Build history of the part. All positions in model axes, mm. Face numbers are marked on the shaded views. A direction names the side the tool comes from. Coordinates: 2 decimals unless noted, no trailing zeros. Order: outer loops, then holes, each group sorted by start corner. A loop starts at its lowest first (then second) coordinate and runs counter-clockwise, first axis right, second up. Notation, with made-up numbers: M 52.25,9 L 88.25,9 A18 ccw 88.25,42 Z; hole C 32.5,9 d1. An arc over 180 degrees is marked long. Write item = value, one per line. Start each with the question number.
Q1. Band-saw the part on D-D on z = 19. Write the cut outline in (x, y), plus the area to 3 significant figures.
Q2. Pull direction Y, two halves, no side cores. Call the marked faces 1, 2 and 3: released by +Y, released by -Y, zero draft, split by the parting line, or undercut.
Q3. 3-axis set-ups, long thin cutter, end or side, ignore diameter. For the marked faces 4, 5 and 6: which of +Z, -Z, +X, -X, +Y, -Y reach the whole face in a straight line?
Q4. Drill centre lines: probe 1 along Y at (x, z) = (21, 53); probe 2 along Y at (x, z) = (12, 86); probe 3 along Y at (x, z) = (22, 88). Where is each one in solid material? Low to high.
Q5. Band-saw the part on C-C on z = 81. Write the cut outline in (x, y), plus the area to 3 significant figures.
Q6. Pin check, flat tips, straight feed: P1, Ø6, axis at x = 24.5, z = 106.5, coming from the +Y side; P2, Ø4, axis at x = 29, y = -279.5, coming from the +Z side; P3, Ø1.5, axis at x = 72.5, y = -75.5, coming from the +Z side. Stop position of each tip, or through.
Q7. Band-saw the part on B-B on z = 128. Write the cut outline in (x, y), plus the area to 3 significant figures.
```python
from build123d import *

# Parameters (mm, degrees)
F1_DEPTH  = 30.48
F3_DEPTH  = 30.48
F5_DEPTH  = 30.48
F6_W      = 152.4
F6_H      = 30.48
F7_DEPTH  = 152.4
F8_W      = 50.8
F8_H      = 127
F9_DEPTH  = 121.92
F11_DEPTH = 475.742
F12_R     = 63.49999


# Not quite as in the source:
# - a fillet or chamfer is up to 0.001 mm smaller than in the source, because OpenCascade refuses the exact size


with BuildPart() as f1:
    # F0 (on Top) → F1 (new body)
    with BuildSketch(Plane.XY):
        Polygon((152.4, 0), (0, 0), (0, -393.7), (50.8, -393.7), align=None)
    extrude(amount=F1_DEPTH)

    # F2 (on face) → F3 (join)
    with BuildSketch(Plane.XY.offset(30.48)):
        Polygon((152.4, -30.48), (152.4, 0), (144.5341935484, -30.48), align=None)
    extrude(amount=-F3_DEPTH)

    # F4 (on face) → F5 (join)
    with BuildSketch(Plane.XY.offset(30.48)):
        Polygon((50.8, -393.7), (152.4, -30.48), (144.5341935484, -30.48), align=None)
    extrude(amount=-F5_DEPTH)

    # F6 (on face) → F7 (join)
    with BuildSketch(Plane.XY.offset(30.48)):
        with Locations((76.2, -15.24)):
            Rectangle(F6_W, F6_H)
    extrude(amount=F7_DEPTH)

    # F8 (on face) → F9 (join)
    with BuildSketch(Plane.XY.offset(30.48)):
        with Locations((25.4, -330.2)):
            Rectangle(F8_W, F8_H)
    extrude(amount=F9_DEPTH)

    # F10 (on face) → F11 (cut)
    with BuildSketch(Plane.YZ.offset(50.8)):
        with BuildLine():
            Line((-330.2, 91.44), (-330.2, 123.19))
            ThreePointArc((-330.2, 123.19), (-352.6506403027, 113.8906403027), (-361.95, 91.44))
            Line((-361.95, 91.44), (-330.2, 91.44))
        make_face()
        with BuildLine():
            ThreePointArc((-298.45, 91.44), (-307.7493596973, 113.8906403027), (-330.2, 123.19))
            Line((-330.2, 123.19), (-330.2, 91.44))
            Line((-330.2, 91.44), (-298.45, 91.44))
        make_face()
        with BuildLine():
            Line((-330.2, 59.69), (-330.2, 91.44))
            Line((-330.2, 91.44), (-361.95, 91.44))
            ThreePointArc((-361.95, 91.44), (-352.6506403027, 68.9893596973), (-330.2, 59.69))
        make_face()
        with BuildLine():
            ThreePointArc((-330.2, 59.69), (-307.7493596973, 68.9893596973), (-298.45, 91.44))
            Line((-298.45, 91.44), (-330.2, 91.44))
            Line((-330.2, 91.44), (-330.2, 59.69))
        make_face()
    extrude(amount=-F11_DEPTH, mode=Mode.SUBTRACT)

    # F12 (radius 63.5 in the source; OpenCascade refuses exactly that, so slightly less here)
    f12_edges = [f1.edges().sort_by_distance(p)[0] for p in [
        (25.4, -393.7, 152.4),
        (25.4, -266.7, 152.4),
    ]]
    fillet(f12_edges, radius=F12_R)


solid = f1.part
```
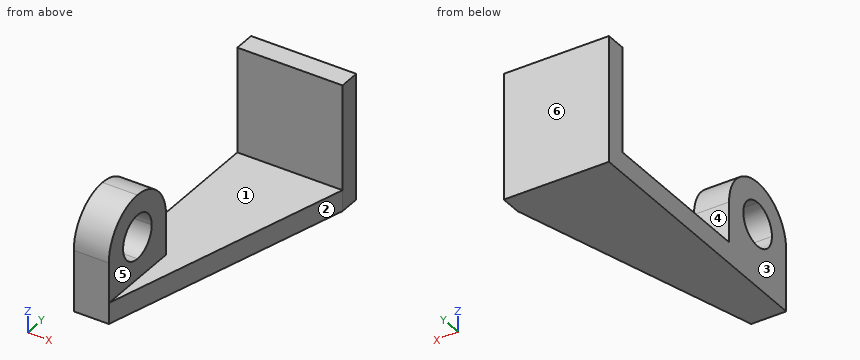
Recorded:
q1.outline = M 0,-393.7 L 50.8,-393.7 L 152.4,-30.48 L 152.4,0 L 0,0 Z
q1.area = 41,500 mm2
q2.face_1 = undercut
q2.face_2 = released by -Y
q2.face_3 = zero draft
q3.face_4 = +Z, +X, -X
q3.face_5 = +Z, +X, -Y
q3.face_6 = +Z, -Z, +X, -X, +Y
q4.probe_1 = -393.7 to -266.7, -30.48 to 0
q4.probe_2 = -393.7 to -361.48, -298.92 to -266.7, -30.48 to 0
q4.probe_3 = -393.7 to -361.76, -298.64 to -266.7, -30.48 to 0
q5.outline = M 0,-393.7 L 50.8,-393.7 L 50.8,-360.18 L 0,-360.18 Z; M 0,-300.22 L 50.8,-300.22 L 50.8,-266.7 L 0,-266.7 Z; M 0,-30.48 L 152.4,-30.48 L 152.4,0 L 0,0 Z
q5.area = 8,050 mm2
q6.P1 = 0
q6.P2 = 129.65
q6.P3 = 30.48
q7.outline = M 0,-380.23 L 50.8,-380.23 L 50.8,-280.17 L 0,-280.17 Z; M 0,-30.48 L 152.4,-30.48 L 152.4,0 L 0,0 Z
q7.area = 9,730 mm2
